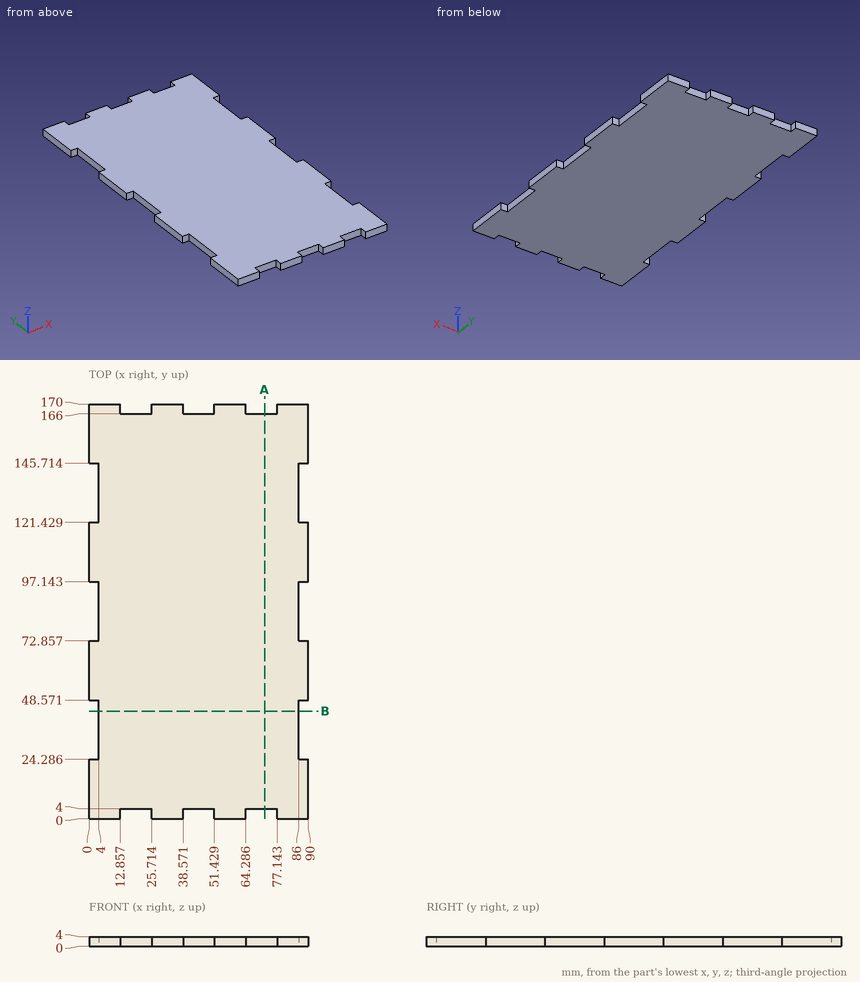
Could you check a few things on this drawing? It's one solid part, dimensions in mm from its lowest x, y, z. Give positions to 0.01 mm unless a question says otherwise; leave off trailing zeros. Loops run counter-clockwise (first coordinate to the right, second up) from the corner with the lowest first, then second, coordinate; pieces in that order, holes last. Notation, with made-up numbers: (8.25, 5) -> (12.25, 5) arc R16 cw to (12.25, 36) -> close; hole circle Ø3 at (-18, 78.5). An arc over 180 degrees is marked (long way). Use one line per item in the form item = value. Start each with the question number.
1) Imagine slicing it at B-B (y = 44). Please give me the cut outline in (x, z), then the cut area to 3 significant figures.
2) Imagine slicing it at A-A (x = 72). Please give me the cut outline in (y, z).
3) Please list where these lines run through material, in increasing order: line 1 along Y through (x, z) = (39, 2.85); line 2 along X through (y, z) = (145.5, 0.65).
4) For P1, Ø2, axis at x = 77, z = 1, coming from the -Y side; P2, Ø2, axis at y = 38.5, z = 1, coming from the -X side; P3, Ø1.2, axis at x = 46, z = 1, coming from the +Y side; P4, Ø1.5, axis at x = 41.5, z = 1, coming from the -Y side, each with a flat end and sliding along its axis, tell me the tip position at first contact or that it passes through.
Check values:
q1.outline = (4, 0) -> (86, 0) -> (86, 4) -> (4, 4) -> close
q1.area = 328 mm^2
q2.outline = (4, 0) -> (166, 0) -> (166, 4) -> (4, 4) -> close
q3.line_1 = 4 to 166
q3.line_2 = 4 to 86
q4.P1 = 0
q4.P2 = 4
q4.P3 = 166
q4.P4 = 4
